CAD build for the part. Positions are in the model's coordinates, mm. Face numbers are marked on the shaded views. A direction names the side the tool comes from. Coordinates: 2 decimals unless noted, no trailing zeros. Loops run counter-clockwise (first coordinate to the right, second up) from the corner with the lowest first, then second, coordinate; pieces in that order, holes last. Notation, with made-up numbers: (-36, -35) -> (5, -35) arc R22 ccw to (5, -2) -> close; hole circle Ø5 at (68.5, 25.5). An arc over 180 degrees is marked (long way). Write item = value, one per line. Start each with the question number.
(1) Band-saw the part on D-D (y = 33.5). Write the cut outline in (x, z).
(2) Band-saw the part on A-A (y = 73.66). Write the cut outline in (x, z), and give its area (3 significant figures).
(3) Flat gauge pins, fed straight in: P1, Ø11, axis at y = 49.21, z = -1.52, coming from the -X side; P2, Ø6, axis at x = 4, y = -22.5, coming from the +Z side; P3, Ø10, axis at y = 3, z = 20, coming from the +X side. Where does each tip first touch, or does it go through?
(4) Pull direction Y, two halves, no side cores. Call the marked faces 4, 5 and 6: +Y half, -Y half, draft (parallel to the pull), parting line (faces both ways), or undercut.
(5) Drill centre lines: line 1 (Y direction, x = 6, z = -2); line 2 (Y direction, x = 5.25, z = -7.5); line 3 (Y direction, x = 0, z = -11). Where is each one in solid material? Low to high. Write a range as from..to.
(6) Tool access for the marked faces 1, 2 and 3: list every direction of +Z, -Z, +X, -X, +Y, -Y with a clear straight run to the whole face (end or side of a thin tool).
(7) Band-saw the part on C-C (x = 2.5). Write the cut outline in (y, z) (3 decimals), and give its area (3 significant figures).
(8) Band-saw the part on B-B (z = 18.5). Write the cut outline in (x, y) (3 decimals), and give its area (3 significant figures).
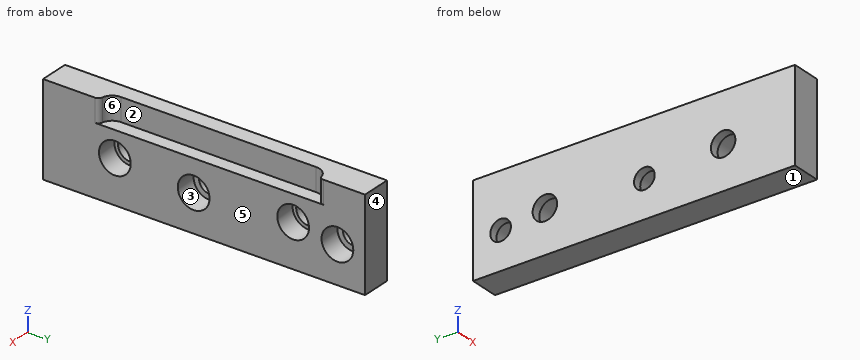
```python
from build123d import *

# Parameters (mm, degrees)
SKETCH1_W           = 16.2814
SKETCH1_H           = 177.8
BOSS_EXTRUDE1_DEPTH = 25.4
SKETCH2_R           = 6.75767
CUT_EXTRUDE1_DEPTH  = 94.879997795
SKETCH3_R           = 8.7641176
CUT_EXTRUDE2_DEPTH  = 11.3284
CUT_EXTRUDE3_DEPTH  = 12.7
SKETCH5_R           = 5.715
CUT_EXTRUDE4_DEPTH  = 94.879997795
SKETCH6_R           = 8.763
CUT_EXTRUDE5_DEPTH  = 11.684
FILLET1_R           = 2.54


with BuildPart() as part:
    # Sketch1 → Boss-Extrude1 (new, symmetric)
    with BuildSketch(Plane.XY):
        Rectangle(SKETCH1_W, SKETCH1_H)
    extrude(amount=BOSS_EXTRUDE1_DEPTH, both=True)

    # Sketch2 → Cut-Extrude1 (cut, through all)
    with BuildSketch(Plane(origin=(8.1407, 0, 0), x_dir=(0, 0, -1), z_dir=(1, 0, 0))):
        with Locations((1.524, 49.211738)):
            Circle(SKETCH2_R)
        with Locations((1.524, -49.211738)):
            Circle(SKETCH2_R)
    extrude(amount=-CUT_EXTRUDE1_DEPTH, mode=Mode.SUBTRACT)

    # Sketch3 → Cut-Extrude2 (cut)
    with BuildSketch(Plane(origin=(8.1407, 0, 0), x_dir=(0, 0, -1), z_dir=(1, 0, 0))):
        with Locations((1.524, 49.211738)):
            Circle(SKETCH3_R)
        with Locations((1.524, -49.211738)):
            Circle(SKETCH3_R)
    extrude(amount=-CUT_EXTRUDE2_DEPTH, mode=Mode.SUBTRACT)

    # Sketch4 → Cut-Extrude3 (cut)
    with BuildSketch(Plane.XY.offset(25.4)):
        with BuildLine():
            Line((0.7493, -51.381727108), (0.7493, 56.38057714))
            ThreePointArc((0.7493, 56.38057714), (2.915188991, 61.601284707), (8.1407, 63.755558905))
            Line((8.1407, 63.755558905), (8.1407, -57.749786229))
            ThreePointArc((8.1407, -57.749786229), (2.985440135, -56.259866378), (0.7493, -51.381727108))
        make_face()
    extrude(amount=-CUT_EXTRUDE3_DEPTH, mode=Mode.SUBTRACT)

    # Sketch5 → Cut-Extrude4 (cut, through all)
    with BuildSketch(Plane(origin=(8.1407, 0, 0), x_dir=(0, 0, -1), z_dir=(1, 0, 0))):
        with Locations((4.7498, -5.715)):
            Circle(SKETCH5_R)
        with Locations((4.7498, 73.66)):
            Circle(SKETCH5_R)
    extrude(amount=-CUT_EXTRUDE4_DEPTH, mode=Mode.SUBTRACT)

    # Sketch6 → Cut-Extrude5 (cut)
    with BuildSketch(Plane(origin=(8.1407, 0, 0), x_dir=(0, 0, -1), z_dir=(1, 0, 0))):
        with Locations((4.7498, -5.715)):
            Circle(SKETCH6_R)
        with Locations((4.7498, 73.66)):
            Circle(SKETCH6_R)
    extrude(amount=-CUT_EXTRUDE5_DEPTH, mode=Mode.SUBTRACT)

    # Fillet1
    fillet1_edges = [part.edges().sort_by_distance(p)[0] for p in [
        (8.1407, -57.749786229, 19.05),
        (8.1407, 63.755558905, 19.05),
    ]]
    fillet(fillet1_edges, radius=FILLET1_R)


solid = part.part
```
Findings below:
q1.outline = (-8.14, -25.4) -> (8.14, -25.4) -> (8.14, 12.7) -> (0.75, 12.7) -> (0.75, 25.4) -> (-8.14, 25.4) -> close
q2.outline = (-8.14, -25.4) -> (8.14, -25.4) -> (8.14, -13.51) -> (-3.54, -13.51) -> (-3.54, -10.46) -> (-8.14, -10.46) -> close; (-8.14, 0.97) -> (-3.54, 0.97) -> (-3.54, 4.01) -> (8.14, 4.01) -> (8.14, 25.4) -> (-8.14, 25.4) -> close
q2.area = 570 mm²
q3.P1 = through
q3.P2 = 12.7
q3.P3 = 0.75
q4.face_4 = +Y half
q4.face_5 = draft
q4.face_6 = undercut
q5.line_1 = -88.9..-57.96, -40.46..-14.04, 2.61..40.46, 57.96..65.34, 81.98..88.9
q5.line_2 = -88.9..-55.62, -42.8..-14.04, 2.61..42.8, 55.62..65.34, 81.98..88.9
q5.line_3 = -88.9..-11.86, 0.43..67.52, 79.8..88.9
q6.face_1 = -Z, +X, -X, +Y, -Y
q6.face_2 = +Z, +X
q6.face_3 = +X
q7.outline = (-88.9, -25.4) -> (88.9, -25.4) -> (88.9, 25.4) -> (61.151, 25.4) -> (61.151, 12.7) -> (-55.795, 12.7) -> (-55.795, 25.4) -> (-88.9, 25.4) -> close; hole circle Ø17.528 at (-49.212, -1.524); hole circle Ø17.526 at (-5.715, -4.75); hole circle Ø17.528 at (49.212, -1.524); hole circle Ø17.526 at (73.66, -4.75)
q7.area = 6,580 mm²
q8.outline = (-8.141, -88.9) -> (8.141, -88.9) -> (8.141, -60.219) arc R2.54 ccw to (6.05, -57.719) arc R6.439 cw to (0.749, -51.382) -> (0.749, 56.381) arc R7.375 cw to (6.247, 63.513) arc R2.54 ccw to (8.141, 65.969) -> (8.141, 88.9) -> (-8.141, 88.9) -> close
q8.area = 2,010 mm²
